Verification items for the finished model (mm, model axes). Face numbers are marked on the shaded views. A direction names the side the tool comes from. Round coordinates to 2 decimals unless told otherwise and drop trailing zeros. Loops run counter-clockwise (first coordinate to the right, second up) from the corner with the lowest first, then second, coordinate; pieces in that order, holes last. Notation, with made-up numbers: (-30, -26) -> (25, -26) arc R22 cw to (25, 3) -> close; hole circle Ø4 at (-19, 6). An arc over 180 degrees is marked (long way). Use a Markdown table: item, result. Add a question column.
Autodesk Inventor part; units mm, degrees
ref_plane "Work Plane1" through (0, 15, 37.0055) normal (0, 0, 1) x (1, 0, 0)
ref_plane "YZ Plane" through (0, 0, 0) normal (1, 0, 0) x (0, 1, 0)
ref_plane "XZ Plane" through (0, 0, 0) normal (0, 1, 0) x (-1, 0, 0)
sketch "Sketch1" plane through (0, 0, 0) normal (0, 1, 0) x (-1, 0, 0)
  circle A0 centre (0, 0) radius 37.0055
  circle A1 centre (0, 0) radius 29.8875
extrude "Extrusion1" add sketch "Sketch1" along normal blind 15 contours A0 | A1
sketch "Sketch2" plane through (0, 15, 0) normal (0, 1, 0) x (1, 0, 0)
  circle A0 centre (0, 0) radius 37.0055
  circle A1 centre (0, 0) radius 30.0306
extrude "Extrusion2" cut sketch "Sketch2" against normal blind 15 contours A1
sketch "Sketch3" plane through (0, 15, 0) normal (0, 1, 0) x (1, 0, 0)
  circle A0 centre (0, 0) radius 37.0055
  line L0 (-34.4949, -13.3982) -> (-31.6379, -11.0586)
  line L1 (-31.6379, -11.0586) -> (-31.6379, 12.0839)
  line L2 (-31.6379, 12.0839) -> (-34.4949, 13.3982)
extrude "Extrusion3" cut sketch "Sketch3" against normal blind 15 contours L2 L1 L0 A0 picked at (-33.4271, 0.3418)
sketch "Sketch4" plane through (0, 15, 0) normal (0, 1, 0) x (1, 0, 0)
  arc A0 (-34.4949, -13.3982) -> (-34.4949, 13.3982) centre (0, 0) ccw
  line L0 (-31.6379, -11.0586) -> (-31.6379, 12.0839)
  line L1 (31.575, 12.0839) -> (31.575, -11.0586)
  line L2 (31.575, -11.0586) -> (34.4949, -13.3982)
  line L3 (31.575, 12.0839) -> (34.4949, 13.3982)
extrude "Extrusion4" cut sketch "Sketch4" against normal blind 15
sketch "Sketch5" plane through (0, 15, 0) normal (0, 1, 0) x (1, 0, 0)
  circle A0 centre (0, 0) radius 30.0306
  line L0 (-31.6379, -11.0586) -> (-34.4949, -13.3982)
  arc A1 (-34.4949, -13.3982) -> (34.4949, -13.3982) centre (0, 0) ccw
  line L1 (-31.6379, -11.0586) -> (-31.6379, 12.0839)
  circle A2 centre (0, 0) radius 30.0306
  line L2 (-31.6379, -11.0586) -> (-28.482, -9.519)
  line L3 (0, -37.0055) -> (0.2981, -30.0291)
extrude "Extrusion5" add sketch "Sketch5" along normal blind 50 contours A0 L3 A1 L0 L2
ref_plane "Work Plane1" through (0, 15, 37.0055) normal (0, 0, 1) x (1, 0, 0)
sketch "Sketch6" plane through (0, 15, 37.0055) normal (0, 0, 1) x (1, 0, 0)
  line L0 (0.2981, 0) -> (0.2981, 50)
  line L1 (0.2981, 41.3903) -> (-3.1652, 41.3903)
  line L2 (-3.1652, 41.3903) -> (-3.1652, 36.7258)
  line L3 (-3.1652, 36.7258) -> (-12.8273, 36.7258)
  line L4 (-12.8273, 36.7258) -> (-12.8273, 10.738)
  line L5 (-12.8273, 10.738) -> (-3.1652, 10.738)
  line L6 (-3.1652, 10.738) -> (-3.1652, 6.7398)
  line L7 (-3.1652, 6.7398) -> (0.2981, 6.7398)
  point P0 (0, -15)
extrude "Extrusion6" cut sketch "Sketch6" against normal blind 10
hole "Hole1" at (-3.1652, 23.7389, 33.3666) direction (-1, 0, 0) diameter 1 depth 3 tip angle 118
hole "Hole2" at (-3.1652, 54.058, 33.3666) direction (-1, 0, 0) diameter 1 depth 3 tip angle 118
properties part number "X-axis-gimbal-part"
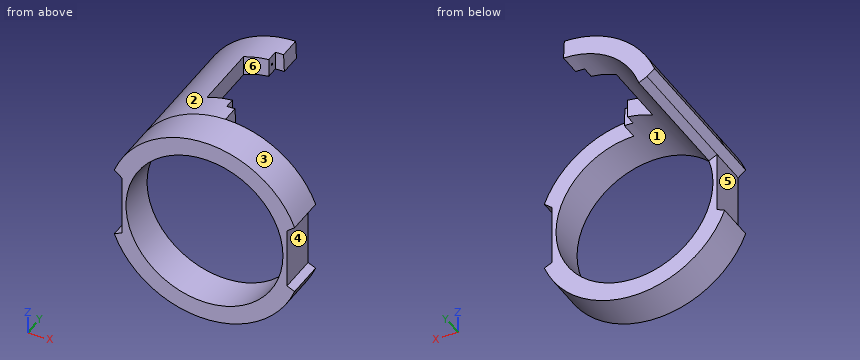
1) Release check for a two-part mould opening along X. For the marked faces 1, 2 and 3 record: released by +X, released by -X, zero draft, split by the parting line, or undercut.
2) Sectioned sample at A-A on z = 0. Enter the section's corners in (x, y) (3 decimals), then the cut area to 3 significant figures.
3) Thickness scan on line 1 (Z direction, x = -0.5, y = 20.5); line 2 (X direction, y = 7, z = 20); line 3 (Y direction, x = 10.5, z = 30). Record the ranges inside material, lowest first.
4) Go/stop test with flat-tipped pins: pin 1 (4 mm diameter, centred on y = 40.5, z = 12.5, fed in from +X); pin 2 (2 mm diameter, centred on y = 33, z = 26, fed in from -X); pin 3 (4.5 mm diameter, centred on y = 9.5, z = -3.5, fed in from -X). Record where each tip stops, or that it passes through.
5) Sectioned sample at B-B on x = -18.5. Enter the section's corners in (y, z), then the cut area to 4 significant figures.
6) Access from +Z, -Z, +X, -X, +Y, -Y to the whole of each face (thin tool, end or side, straight path). Record for the marked faces 4, 5 and 6.
7) Sectioned sample at C-C on y = 27.5. Enter the section's corners in (x, z).
8) Sectioned sample at D-D on y = 13. Enter the section's corners in (x, z) (1 decimal).
Geometry results:
| question | item | result |
|---|---|---|
| 1 | face 1 | undercut |
| 1 | face 2 | released by -X |
| 1 | face 3 | split by the parting line |
| 2 | outline | (-31.638, 0) -> (-30.031, 0) -> (-30.031, 15) -> (-31.638, 15) -> close; (30.031, 0) -> (31.575, 0) -> (31.575, 15) -> (30.031, 15) -> close |
| 2 | area | 47.3 mm^2 |
| 3 | line 1 | 30.03 to 37 |
| 3 | line 2 | -31.14 to -22.4, 22.4 to 31.14 |
| 3 | line 3 | 0 to 15 |
| 4 | pin 1 | x = -26.3 |
| 4 | pin 2 | x = -27.28 |
| 4 | pin 3 | x = -31.64 |
| 5 | outline | (0, -32.05) -> (15, -32.05) -> (15, -23.66) -> (0, -23.66) -> close; (0, 23.66) -> (65, 23.66) -> (65, 32.05) -> (0, 32.05) -> close |
| 5 | area | 671.5 mm^2 |
| 6 | face 4 | +X, +Y, -Y |
| 6 | face 5 | -X, +Y, -Y |
| 6 | face 6 | +Z, -Z, +X |
| 7 | outline | (-34.49, 13.4) -> (-31.64, 11.06) -> (-28.48, 9.52) arc R30.03 cw to (-12.83, 27.15) -> (-12.83, 34.71) arc R37.01 ccw to start |
| 8 | outline | (-34.5, -13.4) arc R37 ccw to (34.5, -13.4) -> (31.6, -12.1) -> (31.6, 11.1) -> (34.5, 13.4) arc R37 ccw to (-34.5, 13.4) -> (-31.6, 11.1) -> (-31.6, -12.1) -> close; hole circle Ø60.1 at (0, 0) |
